```python
from build123d import *

# Parameters (mm, degrees)
SKETCH1_W           = 68
SKETCH1_H           = 15.25
SKETCH1_W_2         = 18
BOSS_EXTRUDE1_DEPTH = 60
SKETCH2_W           = 40
SKETCH2_H           = 15.25
CUT_EXTRUDE1_DEPTH  = 122.264174429
CUT_EXTRUDE2_REACH  = 116.127
CUT_EXTRUDE3_REACH  = 123.264
SKETCH5_R           = 3.25
CUT_EXTRUDE4_REACH  = 105.714
SKETCH6_R           = 2.75
SKETCH7_R           = 2.75
CUT_EXTRUDE5_DEPTH  = 115.127122105
CUT_EXTRUDE6_REACH  = 116.127
SKETCH8_R           = 3.25
SKETCH9_W           = 23
SKETCH9_H           = 21.27
SKETCH9_H_2         = 20
CUT_EXTRUDE7_DEPTH  = 12
CHAMFER1_SIZE       = 1
CUT_EXTRUDE8_REACH  = 123.264
SKETCH10_R          = 3.3
SKETCH10_R_2        = 2.75
SKETCH11_R          = 3.25
CUT_EXTRUDE9_DEPTH  = 125.338248339
CHAMFER2_SIZE       = 1
SKETCH12_W          = 50
SKETCH12_H          = 48
CUT_EXTRUDE10_DEPTH = 5
SKETCH13_W          = 52
SKETCH13_H          = 6
BOSS_EXTRUDE2_DEPTH = 5
SKETCH14_W          = 6
SKETCH14_H          = 32.75
BOSS_EXTRUDE3_DEPTH = 6
SKETCH15_W          = 6
SKETCH15_H          = 15.25
BOSS_EXTRUDE4_DEPTH = 6
BOSS_EXTRUDE5_DEPTH = 10


with BuildPart() as part:
    # Sketch1 → Boss-Extrude1 (new body)
    with BuildSketch(Plane.XY):
        Polygon((0, 0), (-29, 0), (-29, 5), (-5, 5), (-5, 37.75), (-28, 37.75), (-28, 64), (-5, 64), (-5, 76), (18, 76), (18, 64), (73, 64), (73, 0), (52, 0), (52, 5), (68, 5), (68, 37.75), (0, 37.75), align=None)
        with Locations((34, 50.375)):
            Rectangle(SKETCH1_W, SKETCH1_H, mode=Mode.SUBTRACT)
        with Locations((-14, 50.375)):
            Rectangle(SKETCH1_W_2, SKETCH1_H, mode=Mode.SUBTRACT)
    extrude(amount=BOSS_EXTRUDE1_DEPTH)

    # Sketch2 → Cut-Extrude1 (cut, through all)
    with BuildSketch(Plane(origin=(0, 0, 0), x_dir=(0, 0, -1), z_dir=(1, 0, 0))):
        with Locations((-30, 50.375)):
            Rectangle(SKETCH2_W, SKETCH2_H)
    extrude(amount=-CUT_EXTRUDE1_DEPTH, mode=Mode.SUBTRACT)

    # Sketch3 → Cut-Extrude2 (cut, up to next)
    with BuildSketch(Plane(origin=(0, 64, 0), x_dir=(1, 0, 0), z_dir=(0, 1, 0)), mode=Mode.PRIVATE) as cut_extrude2_sk1:
        with BuildLine():
            Line((39.5, -18.5), (46.5, -18.5))
            ThreePointArc((46.5, -18.5), (58, -30), (46.5, -41.5))
            Line((46.5, -41.5), (39.5, -41.5))
            ThreePointArc((39.5, -41.5), (28, -30), (39.5, -18.5))
        make_face()
    cut_extrude2_tool1 = extrude(cut_extrude2_sk1.sketch, amount=-CUT_EXTRUDE2_REACH, mode=Mode.PRIVATE) & part.part
    # Sketch3 → Cut-Extrude2 (cut, up to next)
    with BuildSketch(Plane(origin=(0, 64, 0), x_dir=(1, 0, 0), z_dir=(0, 1, 0)), mode=Mode.PRIVATE) as cut_extrude2_sk2:
        with BuildLine():
            Line((31, -16.25), (24, -16.25))
            ThreePointArc((24, -16.25), (22.25, -14.5), (24, -12.75))
            Line((24, -12.75), (31, -12.75))
            ThreePointArc((31, -12.75), (32.75, -14.5), (31, -16.25))
        make_face()
    cut_extrude2_tool2 = extrude(cut_extrude2_sk2.sketch, amount=-CUT_EXTRUDE2_REACH, mode=Mode.PRIVATE) & part.part
    # Sketch3 → Cut-Extrude2 (cut, up to next)
    with BuildSketch(Plane(origin=(0, 64, 0), x_dir=(1, 0, 0), z_dir=(0, 1, 0)), mode=Mode.PRIVATE) as cut_extrude2_sk3:
        with BuildLine():
            Line((55, -16.25), (62, -16.25))
            ThreePointArc((62, -16.25), (63.75, -14.5), (62, -12.75))
            Line((62, -12.75), (55, -12.75))
            ThreePointArc((55, -12.75), (53.25, -14.5), (55, -16.25))
        make_face()
    cut_extrude2_tool3 = extrude(cut_extrude2_sk3.sketch, amount=-CUT_EXTRUDE2_REACH, mode=Mode.PRIVATE) & part.part
    # Sketch3 → Cut-Extrude2 (cut, up to next)
    with BuildSketch(Plane(origin=(0, 64, 0), x_dir=(1, 0, 0), z_dir=(0, 1, 0)), mode=Mode.PRIVATE) as cut_extrude2_sk4:
        with BuildLine():
            Line((31, -43.75), (24, -43.75))
            ThreePointArc((24, -43.75), (22.25, -45.5), (24, -47.25))
            Line((24, -47.25), (31, -47.25))
            ThreePointArc((31, -47.25), (32.75, -45.5), (31, -43.75))
        make_face()
    cut_extrude2_tool4 = extrude(cut_extrude2_sk4.sketch, amount=-CUT_EXTRUDE2_REACH, mode=Mode.PRIVATE) & part.part
    # Sketch3 → Cut-Extrude2 (cut, up to next)
    with BuildSketch(Plane(origin=(0, 64, 0), x_dir=(1, 0, 0), z_dir=(0, 1, 0)), mode=Mode.PRIVATE) as cut_extrude2_sk5:
        with BuildLine():
            Line((55, -43.75), (62, -43.75))
            ThreePointArc((62, -43.75), (63.75, -45.5), (62, -47.25))
            Line((62, -47.25), (55, -47.25))
            ThreePointArc((55, -47.25), (53.25, -45.5), (55, -43.75))
        make_face()
    cut_extrude2_tool5 = extrude(cut_extrude2_sk5.sketch, amount=-CUT_EXTRUDE2_REACH, mode=Mode.PRIVATE) & part.part
    add(cut_extrude2_tool1.solids().sort_by_distance((43, 64, 30))[0], mode=Mode.SUBTRACT)
    add(cut_extrude2_tool2.solids().sort_by_distance((27.5, 64, 14.5))[0], mode=Mode.SUBTRACT)
    add(cut_extrude2_tool3.solids().sort_by_distance((58.5, 64, 14.5))[0], mode=Mode.SUBTRACT)
    add(cut_extrude2_tool4.solids().sort_by_distance((27.5, 64, 45.5))[0], mode=Mode.SUBTRACT)
    add(cut_extrude2_tool5.solids().sort_by_distance((58.5, 64, 45.5))[0], mode=Mode.SUBTRACT)

    # Sketch5 → Cut-Extrude3 (cut, up to next)
    with BuildSketch(Plane(origin=(0, 76, 0), x_dir=(1, 0, 0), z_dir=(0, 1, 0)), mode=Mode.PRIVATE) as cut_extrude3_sk1:
        with Locations(Location((9, -17.27, 0), (0, 0, 180))):
            Circle(SKETCH5_R)
    cut_extrude3_tool1 = extrude(cut_extrude3_sk1.sketch, amount=-CUT_EXTRUDE3_REACH, mode=Mode.PRIVATE) & part.part
    add(cut_extrude3_tool1.solids().sort_by_distance((9, 76, 17.27))[0], mode=Mode.SUBTRACT)

    # Sketch6 → Cut-Extrude4 (cut, up to next)
    with BuildSketch(Plane(origin=(0, 42.75, 0), x_dir=(1, 0, 0), z_dir=(0, 1, 0)), mode=Mode.PRIVATE) as cut_extrude4_sk1:
        with Locations(Location((9, -17.27, 0), (0, 0, 270))):
            Circle(SKETCH6_R)
    cut_extrude4_tool1 = extrude(cut_extrude4_sk1.sketch, amount=-CUT_EXTRUDE4_REACH, mode=Mode.PRIVATE) & part.part
    add(cut_extrude4_tool1.solids().sort_by_distance((9, 42.75, 17.27))[0], mode=Mode.SUBTRACT)

    # Sketch7 → Cut-Extrude5 (cut, through all)
    with BuildSketch(Plane(origin=(0, 64, 0), x_dir=(1, 0, 0), z_dir=(0, 1, 0))):
        with Locations(Location((-14, -30, 0), (0, 0, 270))):
            Circle(SKETCH7_R)
    extrude(amount=-CUT_EXTRUDE5_DEPTH, mode=Mode.SUBTRACT)

    # Sketch8 → Cut-Extrude6 (cut, up to next)
    with BuildSketch(Plane(origin=(0, 64, 0), x_dir=(1, 0, 0), z_dir=(0, 1, 0)), mode=Mode.PRIVATE) as cut_extrude6_sk1:
        with Locations(Location((-14, -30, 0), (0, 0, 270))):
            Circle(SKETCH8_R)
    cut_extrude6_tool1 = extrude(cut_extrude6_sk1.sketch, amount=-CUT_EXTRUDE6_REACH, mode=Mode.PRIVATE) & part.part
    add(cut_extrude6_tool1.solids().sort_by_distance((-14, 64, 30))[0], mode=Mode.SUBTRACT)

    # Sketch9 → Cut-Extrude7 (cut)
    with BuildSketch(Plane(origin=(0, 76, 0), x_dir=(1, 0, 0), z_dir=(0, 1, 0))):
        with Locations((6.5, -10.635)):
            Rectangle(SKETCH9_W, SKETCH9_H)
        with Locations((6.5, -50)):
            Rectangle(SKETCH9_W, SKETCH9_H_2)
    extrude(amount=-CUT_EXTRUDE7_DEPTH, mode=Mode.SUBTRACT)

    # Chamfer1
    # the kernel refuses this chamfer: 1 mm, written as the material it takes off along each edge
    with BuildSketch(Plane(origin=(-14, 64, 30), x_dir=(0, 0, 1), z_dir=(-1, 0, 0))) as chamfer1_piece_1:
        Polygon((3.25 + CHAMFER1_SIZE, 0), (3.25, -CHAMFER1_SIZE), (3.25, 0), align=None)
    revolve(axis=Axis((-14, 64, 30), (0, 1, 0)), mode=Mode.SUBTRACT)
    with BuildSketch(Plane(origin=(9, 64, 17.27), x_dir=(-1, 0, 0), z_dir=(0, 0, -1))) as chamfer1_piece_2_section:
        Polygon((3.25 + CHAMFER1_SIZE, 0), (3.25, -CHAMFER1_SIZE), (3.25, 0), align=None)
    chamfer1_piece_2 = revolve(axis=Axis((9, 64, 17.27), (0, 1, 0)), mode=Mode.PRIVATE)
    chamfer1_piece_2 = split(chamfer1_piece_2, bisect_by=Plane(origin=(12.733674615, 63.516325385, 21.27), z_dir=(0, 0, -1)), keep=Keep.TOP, mode=Mode.PRIVATE)
    add(chamfer1_piece_2, mode=Mode.SUBTRACT)

    # Sketch10 → Cut-Extrude8 (cut, up to next)
    with BuildSketch(Plane.XZ, mode=Mode.PRIVATE) as cut_extrude8_sk1:
        with Locations((-21, 45)):
            Circle(SKETCH10_R)
    cut_extrude8_tool1 = extrude(cut_extrude8_sk1.sketch, amount=-CUT_EXTRUDE8_REACH, mode=Mode.PRIVATE) & part.part
    # Sketch10 → Cut-Extrude8 (cut, up to next)
    with BuildSketch(Plane.XZ, mode=Mode.PRIVATE) as cut_extrude8_sk2:
        with Locations((-21, 15)):
            Circle(SKETCH10_R)
    cut_extrude8_tool2 = extrude(cut_extrude8_sk2.sketch, amount=-CUT_EXTRUDE8_REACH, mode=Mode.PRIVATE) & part.part
    # Sketch10 → Cut-Extrude8 (cut, up to next)
    with BuildSketch(Plane.XZ, mode=Mode.PRIVATE) as cut_extrude8_sk3:
        with Locations((60, 15)):
            Circle(SKETCH10_R_2)
    cut_extrude8_tool3 = extrude(cut_extrude8_sk3.sketch, amount=-CUT_EXTRUDE8_REACH, mode=Mode.PRIVATE) & part.part
    # Sketch10 → Cut-Extrude8 (cut, up to next)
    with BuildSketch(Plane.XZ, mode=Mode.PRIVATE) as cut_extrude8_sk4:
        with Locations((60, 45)):
            Circle(SKETCH10_R_2)
    cut_extrude8_tool4 = extrude(cut_extrude8_sk4.sketch, amount=-CUT_EXTRUDE8_REACH, mode=Mode.PRIVATE) & part.part
    add(cut_extrude8_tool1.solids().sort_by_distance((-21, 0, 45))[0], mode=Mode.SUBTRACT)
    add(cut_extrude8_tool2.solids().sort_by_distance((-21, 0, 15))[0], mode=Mode.SUBTRACT)
    add(cut_extrude8_tool3.solids().sort_by_distance((60, 0, 15))[0], mode=Mode.SUBTRACT)
    add(cut_extrude8_tool4.solids().sort_by_distance((60, 0, 45))[0], mode=Mode.SUBTRACT)

    # Sketch11 → Cut-Extrude9 (cut, through all)
    with BuildSketch(Plane.ZY.offset(5)):
        with Locations(Location((30.635, 70, 0), (0, 0, 270))):
            Circle(SKETCH11_R)
    extrude(amount=-CUT_EXTRUDE9_DEPTH, mode=Mode.SUBTRACT)

    # Chamfer2
    chamfer2_edges = [part.edges().sort_by_distance(p)[0] for p in [
        (-5, 73.25, 30.635),
    ]]
    chamfer(chamfer2_edges, length=CHAMFER2_SIZE)

    # Sketch12 → Cut-Extrude10 (cut)
    with BuildSketch(Plane(origin=(0, 42.75, 0), x_dir=(1, 0, 0), z_dir=(0, 1, 0))):
        with Locations((43, -30)):
            Rectangle(SKETCH12_W, SKETCH12_H)
    extrude(amount=-CUT_EXTRUDE10_DEPTH, mode=Mode.SUBTRACT)

    # Sketch13 → Boss-Extrude2 (add)
    with BuildSketch(Plane.XZ):
        with Locations((26, 57)):
            Rectangle(SKETCH13_W, SKETCH13_H)
        with Locations((26, 3)):
            Rectangle(SKETCH13_W, SKETCH13_H)
    extrude(amount=-BOSS_EXTRUDE2_DEPTH)

    # Sketch14 → Boss-Extrude3 (add)
    with BuildSketch(Plane.XY.offset(60)):
        with Locations((34, 21.375)):
            Rectangle(SKETCH14_W, SKETCH14_H)
    boss_extrude3 = extrude(amount=-BOSS_EXTRUDE3_DEPTH)

    # Sketch15 → Boss-Extrude4 (add)
    with BuildSketch(Plane.XY.offset(60)):
        with Locations((43, 50.375)):
            Rectangle(SKETCH15_W, SKETCH15_H)
    boss_extrude4 = extrude(amount=-BOSS_EXTRUDE4_DEPTH)

    # Mirror1: Boss-Extrude3, Boss-Extrude4 across plane
    add(boss_extrude3.mirror(Plane.XY.offset(30)))
    add(boss_extrude4.mirror(Plane.XY.offset(30)))

    # Sketch16 → Boss-Extrude5 (add)
    with BuildSketch(Plane.XY.offset(60)):
        Polygon((-28, 37.75), (-5, 14.75), (-5, 37.75), align=None)
    extrude(amount=-BOSS_EXTRUDE5_DEPTH)


solid = part.part
```
Source: CAD feature listing. Evaluate the final solid. Frame: model axes, mm. A direction names the side the tool comes from. Give positions to 0.01 mm unless a question says otherwise; leave off trailing zeros. Write each loop counter-clockwise with the first axis right and the second up, starting at its lowest first coordinate (ties: lowest second). Pieces come first, ordered by that corner, then holes. Notation, with made-up numbers: (52.5, -34.75) - (79.5, -34.75) arc R4 cw to (79.5, -28.75) - close; hole circle Ø11 at (55, 44). An arc over 180 degrees is marked (long way). One line per item, written item: value. Start each with the question number.
Q1. Material intervals for probe 1 along X at (y, z) = (39.2, 30); probe 2 along Y at (x, z) = (-12, 17); probe 3 along X at (y, z) = (40.2, 17.27), sorted ascending. Write a range as from..to.
Q2. Set-up query: faces 4 (the face through (57, 42.75, 3)), 5 (the face through (32.75, 61.04, 14.46)), 6 (the face through (63.75, 61.04, 14.54)), 7 (the face through (52, 2, 30)). Return all of +Z, -Z, +X, -X, +Y, -Y with unobstructed straight access to the full face (end or side cutting, diameter ignored); none if empty.
Q3. Draft query along X for faces 1 (the face through (58, 61, 30)), 2 (the face through (-16.66, 26.41, 55.07)), 3 (the face through (18, 73, 28)). Return one class per face: +X half, -X half, draft (parallel to the pull), parting line (faces both ways), or undercut.
Q4. Section query D-D, the plane x = -21. Return the cut outline in (y, z).
Q5. First-contact query: pin 1 Ø1.8 at (y, z) = (22, 56) entering from -X; pin 2 Ø10 at (x, z) = (-10.5, 49) entering from +Y; pin 3 Ø1 at (y, z) = (61, 16.5) entering from -X. Flat tips, straight axial feed; report the tip coordinate or a pass-through.
Q6. Section query A-A, the plane y = 25.5. Return the cut outline in (x, z), then the cut area to 4 significant figures.
Q7. Section query B-B, the plane x = 9. Count the separate pieces of the cut face and the enclosed holes in it, then the cut area to 3 significant figures.
Q8. Section query C-C, the plane y = 47.5. Return the cut outline in (x, z), then the cut area to 3 significant figures.
Answer:
1. probe 1: x = -28..-16.75, -11.25..18, 68..73
1. probe 2: y = 0..5, 37.75..42.75, 58..64
1. probe 3: x = -28..6.25, 11.75..18, 68..73
2. face 4: +Z, -Z
2. face 5: +Y, -Y
2. face 6: +Y
2. face 7: -Y
3. face 1: undercut
3. face 2: -X half
3. face 3: +X half
4. outline: (0, 0) - (5, 0) - (5, 11.7) - (0, 11.7) - close; (0, 18.3) - (5, 18.3) - (5, 41.7) - (0, 41.7) - close; (0, 48.3) - (5, 48.3) - (5, 60) - (0, 60) - close; (30.75, 50) - (37.75, 50) - (37.75, 0) - (42.75, 0) - (42.75, 60) - (30.75, 60) - close; (58, 0) - (64, 0) - (64, 60) - (58, 60) - close
5. pin 1: stops at x = -13.15
5. pin 2: stops at y = 64
5. pin 3: stops at x = -28
6. outline: (-15.75, 50) - (-5, 50) - (-5, 0) - (0, 0) - (0, 60) - (-15.75, 60) - close; (31, 0) - (37, 0) - (37, 6) - (31, 6) - close; (31, 54) - (37, 54) - (37, 60) - (31, 60) - close; (68, 0) - (73, 0) - (73, 60) - (68, 60) - close
6. area: 779.5 mm2
7. separate pieces: 6
7. enclosed holes: 1
7. area: 844 mm2
8. outline: (-28, 0) - (-23, 0) - (-23, 10) - (-28, 10) - close; (-28, 50) - (-23, 50) - (-23, 60) - (-28, 60) - close; (-5, 0) - (0, 0) - (0, 10) - (-5, 10) - close; (-5, 50) - (0, 50) - (0, 60) - (-5, 60) - close; (40, 0) - (46, 0) - (46, 6) - (40, 6) - close; (40, 54) - (46, 54) - (46, 60) - (40, 60) - close; (68, 0) - (73, 0) - (73, 60) - (68, 60) - close
8. area: 572 mm2
